Can you work these out from the model? Positions are in its coordinate system, mm. Face numbers are marked on the shaded views. A direction names the side the tool comes from. Coordinates: 2 decimals unless noted, no trailing zeros. Loops run counter-clockwise (first coordinate to the right, second up) from the corner with the lowest first, then second, coordinate; pieces in that order, holes last. Notation, with made-up numbers: (63.5, 46.25) -> (88.5, 46.25) arc R24 ccw to (88.5, 78.25) -> close; hole circle Ø6 at (74, -1.5). An arc over 180 degrees is marked (long way). Put each result on its own line as item: value. Start each with the question number.
Item 1: If we section it at A-A on z = 23.5: Please give me the cut outline in (x, y), plus the area to 3 significant figures.
Item 2: If we section it at C-C on y = 23: Please give me the cut outline in (x, z), plus the area to 3 significant figures.
Item 3: If we section it at D-D on x = 12.5: Please give me the cut outline in (y, z).
Item 4: If we section it at B-B on x = 52.5: Please give me the cut outline in (y, z).
Item 5: Please list where these lines run through material, in increasing order: L1, parallel to X at y = 10.5, z = 19.5; L2, parallel to Y at x = 52.5, z = 19.5; L3, parallel to X at y = 9, z = 12. Write a range as from..to.
Item 6: We'd pull the mould along X, two halves only. Please class the marked faces 3, 4 and 5: pulls with the +X half, pulls with the -X half, needs draft (parallel to the pull), parting line crosses it, or undercut.
Item 7: Will these pins go through, and if not, where does the flat tip stop? P1, Ø12, axis at x = -10.5, z = 36, coming from the +Y side; P2, Ø10, axis at y = 26, z = 44, coming from the -X side; P3, Ø12, axis at y = 37, z = 25, coming from the -X side; P4, Ø6, axis at y = 30.5, z = 26, coming from the -X side.
Item 8: For the marked faces 1 and 2, which set-ups out of +Z, -Z, +X, -X, +Y, -Y let a thin tool reach every point of the face, with its end or its side?
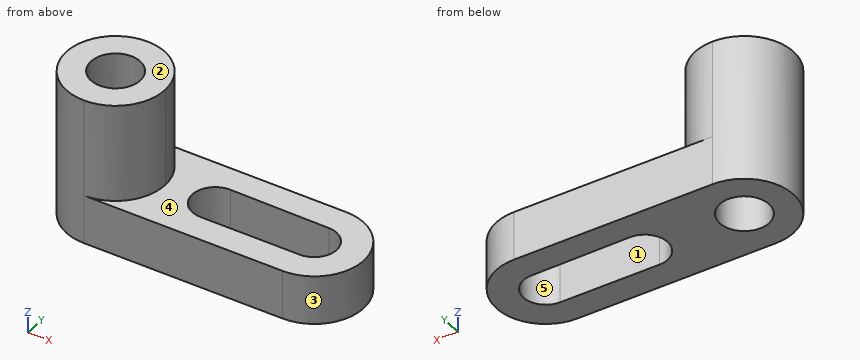
```python
from build123d import *

# Parameters (mm, degrees)
F1_DEPTH = 25.4
F0_R     = 12.7
F2_DEPTH = 76.2


with BuildPart() as f1:
    # F0 (on Top) → F1 (new body)
    with BuildSketch(Plane.XY):
        with BuildLine():
            Line((54.049923, 44.59002), (-47.550077, 44.59002))
            ThreePointArc((-47.550077, 44.59002), (-29.589565, 37.150532), (-22.150077, 19.19002))
            ThreePointArc((-22.150077, 19.19002), (-29.589565, 1.229507), (-47.550077, -6.20998))
            Line((-47.550077, -6.20998), (54.049923, -6.20998))
            ThreePointArc((54.049923, -6.20998), (79.449923, 19.19002), (54.049923, 44.59002))
        make_face()
        with BuildLine():
            Line((3.252867, 31.34379), (54.049923, 30.796887))
            ThreePointArc((54.049923, 30.796887), (65.457669, 19.265659), (54.049923, 7.734431))
            Line((54.049923, 7.734431), (3.252867, 7.734431))
            ThreePointArc((3.252867, 7.734431), (-8.679591, 19.53911), (3.252867, 31.34379))
        make_face(mode=Mode.SUBTRACT)
    extrude(amount=F1_DEPTH)

    # F0 (on Top) → F2 (join)
    with BuildSketch(Plane.XY):
        with BuildLine():
            ThreePointArc((-22.150077, 19.19002), (-29.589565, 37.150532), (-47.550077, 44.59002))
            ThreePointArc((-47.550077, 44.59002), (-72.950077, 19.19002), (-47.550077, -6.20998))
            ThreePointArc((-47.550077, -6.20998), (-29.589565, 1.229507), (-22.150077, 19.19002))
        make_face()
        with Locations((-47.550077, 19.19002)):
            Circle(F0_R, mode=Mode.SUBTRACT)
    extrude(amount=F2_DEPTH)


solid = f1.part
```
Solutions:
1. outline: (-47.55, -6.21) -> (54.05, -6.21) arc R25.4 ccw to (54.05, 44.59) -> (-47.55, 44.59) arc R25.4 ccw to start; hole circle Ø25.4 at (-47.55, 19.19); hole (3.25, 7.73) -> (54.05, 7.73) arc R11.53 ccw to (54.05, 30.8) -> (3.25, 31.34) arc R11.81 ccw (long way) to start
1. area: 5,070 mm^2
2. outline: (-72.66, 0) -> (-59.67, 0) -> (-59.67, 76.2) -> (-72.66, 76.2) -> close; (-35.44, 0) -> (-8.16, 0) -> (-8.16, 25.4) -> (-22.44, 25.4) -> (-22.44, 76.2) -> (-35.44, 76.2) -> close; (64.84, 0) -> (79.16, 0) -> (79.16, 25.4) -> (64.84, 25.4) -> close
2. area: 2,710 mm^2
3. outline: (-6.21, 0) -> (7.73, 0) -> (7.73, 25.4) -> (-6.21, 25.4) -> close; (31.24, 0) -> (44.59, 0) -> (44.59, 25.4) -> (31.24, 25.4) -> close
4. outline: (-6.21, 0) -> (7.73, 0) -> (7.73, 25.4) -> (-6.21, 25.4) -> close; (30.81, 0) -> (44.59, 0) -> (44.59, 25.4) -> (30.81, 25.4) -> close
5. L1: -71.42..-56.81, -38.29..-4.47, 61.42..77.92
5. L2: -6.21..7.73, 30.81..44.59
5. L3: -70.82..-55.13, -39.97..-2.19, 59.18..77.32
6. face 3: pulls with the +X half
6. face 4: needs draft
6. face 5: undercut
7. P1: through
7. P2: x = -72.89
7. P3: x = -70.04
7. P4: x = -71.55
8. face 1: +Z, -Z
8. face 2: +Z, +X, -X, +Y, -Y
